from build123d import *

# Parameters (mm, degrees)
SKETCH3_R           = 48
BOSS_EXTRUDE1_DEPTH = 31
SKETCH4_R           = 2
CUT_EXTRUDE1_DEPTH  = 3.5
SKETCH5_R           = 30
BOSS_EXTRUDE2_DEPTH = 2
SKETCH7_R           = 37.5
BOSS_EXTRUDE3_DEPTH = 12.5
SKETCH6_R           = 21
CUT_EXTRUDE3_DEPTH  = 33
CUT_EXTRUDE4_START  = -3.5
SKETCH8_R           = 2
CUT_EXTRUDE4_DEPTH  = 3.5


with BuildPart() as part:
    # Sketch3 → Boss-Extrude1 (new body)
    with BuildSketch(Plane.XY):
        Circle(SKETCH3_R)
    extrude(amount=BOSS_EXTRUDE1_DEPTH)

    # Sketch4 → Cut-Extrude1 (cut)
    with BuildSketch(Plane.XY.offset(31)):
        with Locations((0, 42)):
            Circle(SKETCH4_R)
        with Locations((29.69848481, 29.69848481)):
            Circle(SKETCH4_R)
        with Locations((42, 0)):
            Circle(SKETCH4_R)
        with Locations((29.69848481, -29.69848481)):
            Circle(SKETCH4_R)
        with Locations((0, -42)):
            Circle(SKETCH4_R)
        with Locations((-29.69848481, -29.69848481)):
            Circle(SKETCH4_R)
        with Locations((-42, 0)):
            Circle(SKETCH4_R)
        with Locations((-29.69848481, 29.69848481)):
            Circle(SKETCH4_R)
    extrude(amount=-CUT_EXTRUDE1_DEPTH, mode=Mode.SUBTRACT)

    # Sketch5 → Boss-Extrude2 (add)
    with BuildSketch(Plane.XY.offset(31)):
        Circle(SKETCH5_R)
    extrude(amount=BOSS_EXTRUDE2_DEPTH)

    # Sketch7 → Boss-Extrude3 (add)
    with BuildSketch(Plane(origin=(0, 0, 0), x_dir=(-1, 0, 0), z_dir=(0, 0, -1))):
        Circle(SKETCH7_R)
    extrude(amount=BOSS_EXTRUDE3_DEPTH)

    # Sketch6 → Cut-Extrude3 (cut)
    with BuildSketch(Plane.XY.offset(33)):
        Circle(SKETCH6_R)
    extrude(amount=-CUT_EXTRUDE3_DEPTH, mode=Mode.SUBTRACT)

    # Sketch8 → Cut-Extrude4 (cut)
    with BuildSketch(Plane(origin=(0, 0, 0), x_dir=(-1, 0, 0), z_dir=(0, 0, -1)).offset(CUT_EXTRUDE4_START)):
        with Locations(Location((0, 42, 0), (0, 0, 180))):
            Circle(SKETCH8_R)
        with Locations(Location((29.69848481, 29.69848481, 0), (0, 0, 180))):
            Circle(SKETCH8_R)
        with Locations(Location((42, 0, 0), (0, 0, 180))):
            Circle(SKETCH8_R)
        with Locations(Location((29.69848481, -29.69848481, 0), (0, 0, 180))):
            Circle(SKETCH8_R)
        with Locations(Location((0, -42, 0), (0, 0, 180))):
            Circle(SKETCH8_R)
        with Locations(Location((-29.69848481, -29.69848481, 0), (0, 0, 180))):
            Circle(SKETCH8_R)
        with Locations(Location((-42, 0, 0), (0, 0, 180))):
            Circle(SKETCH8_R)
        with Locations(Location((-29.69848481, 29.69848481, 0), (0, 0, 180))):
            Circle(SKETCH8_R)
    extrude(amount=CUT_EXTRUDE4_DEPTH, mode=Mode.SUBTRACT)


solid = part.part
Source: CAD feature listing. Evaluate the final solid. Frame: model axes, mm. A direction names the side the tool comes from. Coordinates: 2 decimals unless noted, no trailing zeros. Order: outer loops, then holes, each group sorted by start corner. A loop starts at its lowest first (then second) coordinate and runs counter-clockwise, first axis right, second up.
Item 1: Cut plane D-D (z = 24.5). Return loops of the section in (x, y).
Output values:
outline: circle Ø96 at (0, 0); hole circle Ø42 at (0, 0)
Item 2: Cut plane C-C (z = -9.5). Return loops of the section in (x, y).
Output values:
outline: circle Ø75 at (0, 0)
Item 3: Set-up query: faces 1 (the face through (27.7, 29.8, 29.3)), 2 (the face through (28.22, 28.35, 1.77)), 3 (the face through (-47.954, 2.11, 15.283)). Return all of +Z, -Z, +X, -X, +Y, -Y with unobstructed straight access to the full face (end or side cutting, diameter ignored); none if empty.
Output values:
face 1: +Z
face 2: -Z
face 3: +Z, -Z
Item 4: First-contact query: P1, Ø5, axis at y = -20, z = -4.5, coming from the +X side; P2, Ø4.5, axis at x = 29.7, y = -29.7, coming from the +Z side; P3, Ø3, axis at x = -29.7, y = 29.7, coming from the -Z side. Flat tips, straight axial feed; report the tip coordinate or a pass-through.
Output values:
P1: stops at x = 33.17
P2: stops at z = 31
P3: stops at z = 3.5
Item 5: Material intervals for line 1 (Y direction, x = 0, z = 30.2); line 2 (Y direction, x = 0, z = 7); line 3 (Y direction, x = 42.5, z = 0.5), sorted ascending.
Output values:
line 1: y = -48 to -44, -40 to -21, 21 to 40, 44 to 48
line 2: y = -48 to -21, 21 to 48
line 3: y = -22.31 to -1.94, 1.94 to 22.31
Item 6: Pull-direction query (X, two-part tool) for faces 4 (the face through (-30, 30, 27.5)), 5 (the face through (-29.97, 1.32, 31.99)); classes: pulls with the +X half, pulls with the -X half, needs draft (parallel to the pull), parting line crosses it, or undercut.
Output values:
face 4: undercut
face 5: parting line crosses it
